Autodesk Inventor part; units mm, degrees
ref_plane "YZ Plane" through (0, 0, 0) normal (1, 0, 0) x (0, 1, 0)
ref_plane "XZ Plane" through (0, 0, 0) normal (0, 1, 0) x (-1, 0, 0)
ref_plane "XY Plane" through (0, 0, 0) normal (0, 0, 1) x (1, 0, 0)
sketch "Sketch1" plane through (0, 0, 0) normal (0, 0, 1) x (1, 0, 0)
  circle A0 centre (0, 0) radius 70
  circle A1 centre (0, -45) radius 5.25
  circle A2 centre (0, 0) radius 11
  circle A3 centre (6, 47.5) radius 1.55
  circle A4 centre (-6, 47.5) radius 1.55
  circle A5 centre (15.4998, 15.4998) radius 1.5
  circle A6 centre (0, -29) radius 2.5
  circle A7 centre (0, -61) radius 2.5
  circle A8 centre (52.8275, 30.5) radius 2.5
  circle A9 centre (38.9711, 22.5) radius 5.25
  circle A10 centre (25.1147, 14.5) radius 2.5
  circle A11 centre (-52.8275, 30.5) radius 2.5
  circle A12 centre (-38.9711, 22.5) radius 5.25
  circle A13 centre (-25.1147, 14.5) radius 2.5
  circle A14 centre (0, 0) radius 21.92 construction
  circle A15 centre (-15.4998, 15.4998) radius 1.5
  circle A16 centre (-15.4998, -15.4998) radius 1.5
  circle A17 centre (15.4998, -15.4998) radius 1.5
  dimension "d53" = 43.84
  dimension "D_B" = 140
  dimension "Furos" = 10.5
  dimension "d11" = 22
  dimension "d24" = 3.1
  dimension "d25" = 3.1
  dimension "FN" = 3
  dimension "d31" = 5
  dimension "d32" = 5
  dimension "d34" = 16
  dimension "d35" = 16
  dimension "d39" = 47.5
  dimension "d40" = 45
  dimension "d50" = 360
  dimension "d56" = 360
  dimension "d58" = 15.4998
  dimension "d59" = 15.4998
  dimension "d60" = 12
  dimension "d61" = 6
extrude "Extrusion1" add sketch "Sketch1" along normal blind 4
properties part number "Topo"
Verification items for the finished model (mm, model axes). Coordinates: 2 decimals unless noted, no trailing zeros. Order: outer loops, then holes, each group sorted by start corner. A loop starts at its lowest first (then second) coordinate and runs counter-clockwise, first axis right, second up. Notation, with made-up numbers: (61.5, 45.25) - (114.5, 45.25) arc R20 ccw to (114.5, 53.25) - close; hole circle Ø1 at (83.5, 84.5). An arc over 180 degrees is marked (long way). Return JSON: item names as keys, results as strings.
(1) Thickness scan on line 1 along Y through (x, z) = (0, 2.85); line 2 along X through (y, z) = (24, 2.1); line 3 along Y through (x, z) = (16.5, 2.8). Record the ranges inside material, lowest first.
Filled sheet:
{"line 1": "y = -70 to -63.5, -58.5 to -50.25, -39.75 to -31.5, -26.5 to -11, 11 to 70", "line 2": "x = -65.76 to -44, -33.94 to 33.94, 44 to 65.76", "line 3": "y = -68.03 to -16.62, -14.38 to 14.38, 16.62 to 68.03"}
(2) Section check D-D, the plane y = 19.5. Record the cut outline in (x, z).
Filled sheet:
{"outline": "(-67.23, 0) - (-43.28, 0) - (-43.28, 4) - (-67.23, 4) - close; (-34.66, 0) - (34.66, 0) - (34.66, 4) - (-34.66, 4) - close; (43.28, 0) - (67.23, 0) - (67.23, 4) - (43.28, 4) - close"}
(3) Mould release check, pull along Y, two halves, no side actions. Record for faces 1 (the cylindrical face through (-55.55, 42.594, 1.972)), 2 (the cylindrical face through (-14.114, 16.074, 1.972)), 3 (the flat face through (15, 1, 0)): pulls with the +Y half, pulls with the -Y half, needs draft (parallel to the pull), parting line crosses it, or undercut.
Filled sheet:
{"face 1": "parting line crosses it", "face 2": "undercut", "face 3": "needs draft"}
(4) Section check A-A, the plane y = 0. Record the cut outline in (x, z), and give its area (3 significant figures).
Filled sheet:
{"outline": "(-70, 0) - (-11, 0) - (-11, 4) - (-70, 4) - close; (11, 0) - (70, 0) - (70, 4) - (11, 4) - close", "area": "472 mm^2"}
(5) Section check C-C, the plane x = -42.5. Record the cut outline in (y, z).
Filled sheet:
{"outline": "(-55.62, 0) - (18.61, 0) - (18.61, 4) - (-55.62, 4) - close; (26.39, 0) - (55.62, 0) - (55.62, 4) - (26.39, 4) - close"}
(6) Section check B-B, the plane z = 1.8. Give the number of separate pieces and of enclosed holes in the cut face, and give its area (3 significant figures).
Filled sheet:
{"separate pieces": "1", "enclosed holes": "16", "area": "14,600 mm^2"}
(7) Go/stop test with flat-tipped pins: pin 1 (2.5 mm diameter, centred on x = -15.5, y = -15.5, fed in from +Z); pin 2 (1 mm diameter, centred on y = 24.5, z = 0.5, fed in from -X); pin 3 (2 mm diameter, centred on x = -18, z = 1.5, fed in from -Y); pin 4 (1 mm diameter, centred on x = 38, z = 2, fed in from -Y). Record where each tip stops, or that it passes through.
Filled sheet:
{"pin 1": "passes through", "pin 2": "stops at x = -65.76", "pin 3": "stops at y = -67.9", "pin 4": "stops at y = -59.11"}
